from build123d import *

# Parameters (mm, degrees)
SKETCH1_W           = 150
SKETCH1_H           = 150
SKETCH1_R           = 35
BOSS_EXTRUDE1_DEPTH = 10
BOSS_EXTRUDE2_DEPTH = 10


with BuildPart() as part:
    # Sketch1 → Boss-Extrude1 (new body)
    with BuildSketch(Plane(origin=(0, 0, 0), x_dir=(1, 0, 0), z_dir=(0, 1, 0))):
        with Locations((75, -75)):
            Rectangle(SKETCH1_W, SKETCH1_H)
        with Locations(Location((50, -75, 0), (0, 0, 270))):
            Circle(SKETCH1_R, mode=Mode.SUBTRACT)
    extrude(amount=BOSS_EXTRUDE1_DEPTH)

    # Sketch7 → Boss-Extrude2 (add)
    with BuildSketch(Plane(origin=(0, 10, 0), x_dir=(1, 0, 0), z_dir=(0, 1, 0))):
        with BuildLine():
            Line((117.065640108, -19.374526579), (137.010556372, -20.857872537))
            ThreePointArc((137.010556372, -20.857872537), (135, -75), (137.010556372, -129.142127463))
            Line((137.010556372, -129.142127463), (117.065640108, -130.625473421))
            ThreePointArc((117.065640108, -130.625473421), (115, -75), (117.065640108, -19.374526579))
        make_face()
    extrude(amount=BOSS_EXTRUDE2_DEPTH)


solid = part.part
The model under review builds one solid part; all positions refer to its coordinate system, in mm. A direction names the side the tool comes from. Give positions to 0.01 mm unless a question says otherwise; leave off trailing zeros. Order: outer loops, then holes, each group sorted by start corner. A loop starts at its lowest first (then second) coordinate and runs counter-clockwise, first axis right, second up. Notation, with made-up numbers: M -28,58 L 5,58 A16 cw 5,68 Z; hole C 87.5,-26 d4. An arc over 180 degrees is marked long. Answer in a Markdown table with one row per item. Add a question column.
1. To check wall thickness, follow line 1 along X through (y, z) = (3.5, 75); line 2 along Y through (x, z) = (13, 30.5); line 3 along X through (y, z) = (1.75, 49). State the ranges of each line that lie inside material, in increasing order.
2. Add section A-A on x = 50. State the section outline as (y, z) points.
3. Mouldability with a two-part tool opening along Z and no side actions: class faces 1 (the cylindrical face through (84.7, 4.93, 70.44)), 2 (the flat face through (74, 5, 0)), 3 (the cylindrical face through (135, 15, 74)), 4 (the flat face through (150, 5, 76)) as released by +Z, released by -Z, zero draft, split by the parting line, or undercut.
4. Machinability: for faces 5 (the flat face through (126.898, 14.93, 20.106)), 6 (the flat face through (91, 0, 74)), 7 (the flat face through (126, 20, 74)), 8 (the cylindrical face through (115, 15, 76)), 9 (the flat face through (127.178, 14.93, 129.873)), which of the approach directions +Z, -Z, +X, -X, +Y, -Y give a long, thin tool a straight path to every point of the face, cutting with its end or side? Answer none if there is none.
5. Add section D-D on z = 107. State the section outline as (x, y) points.
6. For pin 1 Ø4 at (y, z) = (12.5, 134.5) entering from -X; pin 2 Ø1.5 at (x, z) = (95.5, 122) entering from +Y, all flat-tipped, find the tip position at first contact; note any pin that passes through.
7. Add section B-B on z = 75. State the section outline as (x, y) points.
8. Add section C-C on y = 7. State the section outline as (x, z) points.
The answers:
| question | item | result |
|---|---|---|
| 1 | line 1 | 0 to 15, 85 to 150 |
| 1 | line 2 | 0 to 10 |
| 1 | line 3 | 0 to 26.57, 73.43 to 150 |
| 2 | outline | M 0,0 L 10,0 L 10,40 L 0,40 Z; M 0,110 L 10,110 L 10,150 L 0,150 Z |
| 3 | face 1 | undercut |
| 3 | face 2 | released by -Z |
| 3 | face 3 | undercut |
| 3 | face 4 | zero draft |
| 4 | face 5 | -Z, +X, +Y |
| 4 | face 6 | +Z, -Z, +X, -X, -Y |
| 4 | face 7 | +Z, -Z, +X, -X, +Y |
| 4 | face 8 | -X, +Y |
| 4 | face 9 | +Z, +X, +Y |
| 5 | outline | M 0,0 L 35.82,0 L 35.82,10 L 0,10 Z; M 64.18,0 L 150,0 L 150,10 L 135.7,10 L 135.7,20 L 115.68,20 L 115.68,10 L 64.18,10 Z |
| 6 | pin 1 | through |
| 6 | pin 2 | y = 10 |
| 7 | outline | M 0,0 L 15,0 L 15,10 L 0,10 Z; M 85,0 L 150,0 L 150,10 L 135,10 L 135,20 L 115,20 L 115,10 L 85,10 Z |
| 8 | outline | M 0,0 L 150,0 L 150,150 L 0,150 Z; hole C 50,75 d70 |
